Input: part model. Units: mm. Frame: model coordinates. A direction names the side the tool comes from. Give positions to 0.01 mm unless a question says otherwise; leave off trailing zeros. Loops run counter-clockwise (first coordinate to the right, second up) from the corner with the lowest first, then second, coordinate; pieces in that order, holes last. Notation, with made-up numbers: (70.5, -21) - (113.5, -21) arc R21 cw to (113.5, -10) - close; hole circle Ø3 at (73.5, 62). An arc over 180 degrees is marked (long way). Answer as a JSON object with one key per item and string values. Group by question number.
(1) Material intervals for L1, parallel to Y at x = -8, z = -3.25; L2, parallel to Y at x = -1, z = -1.5 (3 decimals); L3, parallel to Z at x = -5.5, y = -16, sorted ascending.
(2) Section query A-A (y = -5.5). Return loops of the section in (x, z) (3 decimals), plus the area to 3 significant figures.
(3) Pin query (flat end, axial travel): P1, Ø2, axis at y = -10.5, z = -2, coming from the +X side; P2, Ø6, axis at y = -11.5, z = -5, coming from the -X side; P3, Ø4, axis at x = 2.5, z = 0, coming from the +Y side (3 decimals); P4, Ø2, axis at x = -7.5, z = 1, coming from the -Y side. Return the tip coordinate at first contact, or that it passes through.
(4) Access query for faces 1 (the flat face through (0, 0, 5)), 2 (the cylindrical face through (-6.75, -9.658, -6.197)), 3 (the cylindrical face through (1, -24, 0)), 4 (the cylindrical face through (9.525, -9.392, -0.06)), 5 (the flat face through (0, 2, 3.5)). Directions: +Z, -Z, +X, -X, +Y, -Y. A direction counts if a zero-diameter tool reaches every point of the face in a straight line with its end or side. Return the directions, or none.
(5) Section query D-D (y = 0.5). Return loops of the section in (x, z) (1 decimal).
```python
from build123d import *

# Parameters (mm, degrees)
F1_DEPTH  = 19.05
F2_R      = 5.08
F3_R      = 2.5
F4_DEPTH  = 2
F5_R      = 1
F6_DEPTH  = 5
F8_DEPTH  = 3.175
F9_R      = 1
F10_DEPTH = 1
F12_ANGLE = 90


# Not quite as in the source:
# - a length typed as a fraction of an inch, garbled in the dataset ("3 / 203.2 mm" for 3/8 in), is restored


with BuildPart() as f1:
    # F0 (on Top) → F1 (new body)
    with BuildSketch(Plane.XY):
        with BuildLine():
            Line((0, 7), (-6.4595375221, 7))
            ThreePointArc((-6.4595375221, 7), (-9.525, 0), (-6.4595375221, -7))
            Line((-6.4595375221, -7), (6.4595375221, -7))
            ThreePointArc((6.4595375221, -7), (9.525, 0), (6.4595375221, 7))
            Line((6.4595375221, 7), (0, 7))
        make_face()
    extrude(amount=F1_DEPTH)

    # F2
    f2_edges = [f1.edges().sort_by_distance(p)[0] for p in [
        (-6.459538, -7, 9.525),
        (6.459538, -7, 9.525),
        (-6.459538, 7, 9.525),
        (6.459538, 7, 9.525),
    ]]
    fillet(f2_edges, radius=F2_R)

    # F3 (on face) → F4 (join)
    with BuildSketch(Plane.XY.offset(19.05)):
        Circle(F3_R)
    extrude(amount=F4_DEPTH)

    # F5 (on face) → F6 (join)
    with BuildSketch(Plane.XY.offset(21.05)):
        Circle(F5_R)
    extrude(amount=F6_DEPTH)

    # F7 (on face) → F8 (join)
    with BuildSketch(Plane(origin=(0, 0, 0), x_dir=(1, 0, 0), z_dir=(0, 0, -1))):
        with BuildLine():
            Line((0, -3.5), (3.2297687611, -3.5))
            ThreePointArc((3.2297687611, -3.5), (0, 4.7625), (-3.2297687611, -3.5))
            Line((-3.2297687611, -3.5), (0, -3.5))
        make_face()
    extrude(amount=F8_DEPTH)

    # F9 (on face) → F10 (join)
    with BuildSketch(Plane(origin=(0, 0, -3.175), x_dir=(1, 0, 0), z_dir=(0, 0, -1))):
        Circle(F9_R)
    extrude(amount=F10_DEPTH)


with BuildPart() as f1_1:
    # F12: moved
    add(f1.part.rotate(Axis((1.8931087106, 0, 0), (1, 0, 0)), F12_ANGLE))


solid = f1_1.part
```
Recorded:
{
 "1": {"L1": "y = -19.05 to 0", "L2": "y = -21.05 to 3.175", "L3": "z = -6.78 to 6.78"},
 "2": {"outline": "(-8.591, -4.114) arc R5.08 ccw to (-4.009, -7) - (4.009, -7) arc R5.08 ccw to (8.591, -4.114) arc R9.525 ccw to (8.591, 4.114) arc R5.08 ccw to (4.009, 7) - (-4.009, 7) arc R5.08 ccw to (-8.591, 4.114) arc R9.525 ccw to start", "area": "236 mm^2"},
 "3": {"P1": "stops at x = 9.47", "P2": "stops at x = -9.31", "P3": "stops at y = 4.175", "P4": "stops at y = -19.05"},
 "4": {"face 1": "+Y", "face 2": "-Z, -X, +Y, -Y", "face 3": "-Y", "face 4": "+X, +Y, -Y", "face 5": "+Z, +X, -X, +Y"},
 "5": {"outline": "(-3.2, 3.5) arc R4.8 ccw (long way) to (3.2, 3.5) - close"}
}
